Could you check a few things on this model? Use its own coordinates, in mm. Face numbers are marked on the shaded views. Give positions to 0.01 mm unless a question says otherwise; leave off trailing zeros. Loops run counter-clockwise (first coordinate to the right, second up) from the corner with the lowest first, then second, coordinate; pieces in that order, holes last. Notation, with made-up numbers: (33.25, 79) - (71.25, 79) arc R21 ccw to (71.25, 101) - close; hole circle Ø6 at (53.25, 47.5). An arc over 180 degrees is marked (long way). Answer in a Markdown table with one row per item. Add a question column.
```python
from build123d import *

# Parameters (mm, degrees)
F1_DEPTH = 20
F2_R     = 12.7
F3_DEPTH = 3.5
F5_D     = 6


with BuildPart() as f1:
    # F0 (on Front) → F1 (new body)
    with BuildSketch(Plane.XZ):
        Polygon((17.424202, 12.846258), (3.237095, 21.404447), (-12.846258, 17.424202), (-21.404447, 3.237095), (-17.424202, -12.846258), (-3.237095, -21.404447), (12.846258, -17.424202), (21.404447, -3.237095), align=None)
    extrude(amount=F1_DEPTH)

    # F2 (on face) → F3 (cut)
    with BuildSketch(Plane.XZ.offset(20)):
        Circle(F2_R)
    extrude(amount=-F3_DEPTH, mode=Mode.SUBTRACT)

    # F5 (through all)
    with Locations(Plane.XZ.offset(16.5)):
        with Locations((0, 0)):
            Hole(F5_D / 2)


solid = f1.part
```
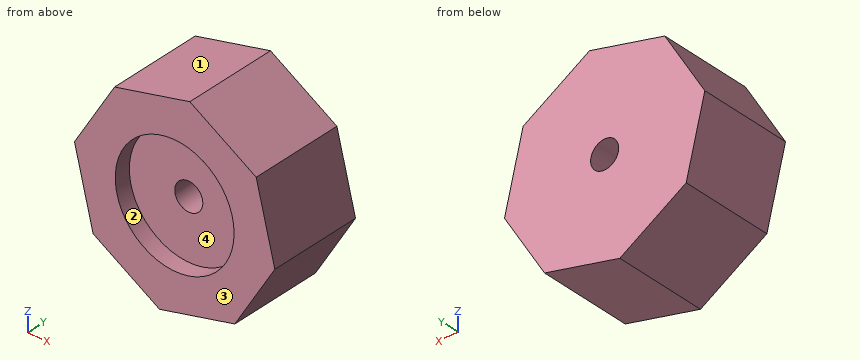
(1) Please list where these lines run through material, in increasing order: line 1 (Y direction, x = -6.5, z = 3); line 2 (Z direction, x = -0.5, y = -12.75); line 3 (Z direction, x = 0, y = -10).
(2) I want a section at A-A on y = -18.5. Please give me the cut outline in (x, z), then the cut area to 3 significant figures.
(3) For pin 1 Ø2 at (y, z) = (-3, -14) entering from -X; pin 2 Ø3 at (y, z) = (-9.5, 11) entering from +X; pin 3 Ø12 at (y, z) = (-3.5, -5.5) entering from -X, each with a flat end and sliding along its axis, tell me the tip position at first contact or that it passes through.
(4) I want a section at D-D on x = 0. Please give me the cut outline in (y, z).
(5) I want a section at C-C on x = -5. Please give me the cut outline in (y, z), then the cut area to 3 significant figures.
(6) I want a section at B-B on z = 1. Please give me the cut outline in (x, y).
(7) We'd pull the mould along X, two halves only. Please class the marked faces 1, 2, 3 and 4: pulls with the +X half, pulls with the -X half, needs draft (parallel to the pull), parting line crosses it, or undercut.
Reported:
| question | item | result |
|---|---|---|
| 1 | line 1 | -16.5 to 0 |
| 1 | line 2 | -20.73 to -2.96, 2.96 to 20.48 |
| 1 | line 3 | -20.6 to -3, 3 to 20.6 |
| 2 | outline | (-21.4, 3.24) - (-17.42, -12.85) - (-3.24, -21.4) - (12.85, -17.42) - (21.4, -3.24) - (17.42, 12.85) - (3.24, 21.4) - (-12.85, 17.42) - close; hole circle Ø25.4 at (0, 0) |
| 2 | area | 819 mm² |
| 3 | pin 1 | x = -17.17 |
| 3 | pin 2 | x = 18.25 |
| 3 | pin 3 | x = -20.73 |
| 4 | outline | (-20, -20.6) - (0, -20.6) - (0, -3) - (-16.5, -3) - (-16.5, -12.7) - (-20, -12.7) - close; (-20, 12.7) - (-16.5, 12.7) - (-16.5, 3) - (0, 3) - (0, 20.6) - (-20, 20.6) - close |
| 5 | outline | (-20, -20.34) - (0, -20.34) - (0, 19.37) - (-20, 19.37) - (-20, 11.67) - (-16.5, 11.67) - (-16.5, -11.67) - (-20, -11.67) - close |
| 5 | area | 712 mm² |
| 6 | outline | (-20.85, -20) - (-12.66, -20) - (-12.66, -16.5) - (-2.83, -16.5) - (-2.83, 0) - (-20.85, 0) - close; (2.83, -16.5) - (12.66, -16.5) - (12.66, -20) - (20.36, -20) - (20.36, 0) - (2.83, 0) - close |
| 7 | face 1 | pulls with the -X half |
| 7 | face 2 | undercut |
| 7 | face 3 | needs draft |
| 7 | face 4 | undercut |
